from build123d import *

# Parameters (mm, degrees)
F0_W      = 5
F0_H      = 370
F1_DEPTH  = 100
F0_W_2    = 20
F0_W_3    = 389
F0_H_2    = 20
F2_DEPTH  = 5
F3_W      = 20
F3_H      = 370
F4_DEPTH  = 5
F3_W_2    = 389
F3_H_2    = 20
F5_DEPTH  = 5
F7_DEPTH  = 20
F8_DEPTH  = 25
F10_DEPTH = 20
F9_W      = 45
F9_H      = 5
F11_DEPTH = 100


with BuildPart() as f1:
    # F0 (on Front) → F1 (new body)
    with BuildSketch(Plane.XZ):
        Polygon((-205.3960859776, 18.3333333333), (-205.3960859776, 13.3333333333), (183.6039140224, 13.3333333333), (183.6039140224, 18.3333333333), (163.6039140225, 18.3333333333), (158.6039140225, 18.3333333333), (-180.3960859776, 18.3333333333), (-185.3960859776, 18.3333333333), align=None)
        with Locations((-182.8960859776, 203.3333333333)):
            Rectangle(F0_W, F0_H)
        with Locations((161.1039140225, 203.3333333333)):
            Rectangle(F0_W, F0_H)
    extrude(amount=F1_DEPTH)

    # F0 (on Front) → F2 (join)
    with BuildSketch(Plane.XZ):
        with Locations((-195.3960859776, 203.3333333333)):
            Rectangle(F0_W_2, F0_H)
        with Locations((-10.8960859776, 3.3333333333)):
            Rectangle(F0_W_3, F0_H_2)
        with Locations((173.6039140224, 203.3333333333)):
            Rectangle(F0_W_2, F0_H)
    extrude(amount=F2_DEPTH)

    # F3 (on face) → F4 (join)
    with BuildSketch(Plane.XZ.offset(100)):
        with Locations((-195.3960859776, 203.3333333333)):
            Rectangle(F3_W, F3_H)
    extrude(amount=-F4_DEPTH)

    # F3 (on face) → F5 (join)
    with BuildSketch(Plane.XZ.offset(100)):
        with Locations((-10.8960859776, 3.3333333333)):
            Rectangle(F3_W_2, F3_H_2)
        with Locations((173.6039140225, 203.3333333333)):
            Rectangle(F3_W, F3_H)
    extrude(amount=-F5_DEPTH)

    # F7 (cut): a face of the model
    f7_faces = [f1.faces().sort_by_distance(p)[0] for p in [
        (162.573137616, -50, 388.3333333333),
    ]]
    extrude(f7_faces, amount=-F7_DEPTH, mode=Mode.SUBTRACT)

    # F6 (on face) → F8 (cut)
    with BuildSketch(Plane.YZ.offset(-180.3960859776)):
        with BuildLine():
            Line((-81.7000014901, 341.2361545223), (-81.7000014901, 320.7823193073))
            Line((-81.7000014901, 320.7823193073), (-53.5750014901, 320.7823193073))
            ThreePointArc((-53.5750014901, 320.7823193073), (-51.7353107636, 325.2108260661), (-47.2992664142, 327.0322663236))
            Line((-47.2992664142, 327.0322663236), (-47.1841779607, 354.9823193073))
            Line((-47.1841779607, 354.9823193073), (-68.0701213982, 354.9823193073))
            ThreePointArc((-68.0701213982, 354.9823193073), (-75.7291590422, 348.9461939299), (-81.7000014901, 341.2361545223))
        make_face()
        with BuildLine():
            ThreePointArc((-81.7000014901, 341.2361545223), (-85.8931230415, 331.3889210251), (-87.3250014901, 320.7823193073))
            Line((-87.3250014901, 320.7823193073), (-81.7000014901, 320.7823193073))
            Line((-81.7000014901, 320.7823193073), (-81.7000014901, 341.2361545223))
        make_face()
        with BuildLine():
            Line((-81.7000014901, 320.7823193073), (-87.3250014901, 320.7823193073))
            ThreePointArc((-87.3250014901, 320.7823193073), (-85.8931230415, 310.1757175895), (-81.7000014901, 300.3284840924))
            Line((-81.7000014901, 300.3284840924), (-81.7000014901, 320.7823193073))
        make_face()
        with BuildLine():
            Line((-13.3000014901, 320.7823193073), (-13.3000014901, 299.7514045626))
            ThreePointArc((-13.3000014901, 299.7514045626), (-8.847735475, 309.8507137528), (-7.3250014901, 320.7823193073))
            ThreePointArc((-7.3250014901, 320.7823193073), (-8.847735475, 331.7139248619), (-13.3000014901, 341.8132340521))
            Line((-13.3000014901, 341.8132340521), (-13.3000014901, 320.7823193073))
        make_face()
        with BuildLine():
            Line((-47.3507365661, 314.5323722911), (-47.4658250195, 286.5823193073))
            Line((-47.4658250195, 286.5823193073), (-26.579881582, 286.5823193073))
            ThreePointArc((-26.579881582, 286.5823193073), (-19.1594603041, 292.3798143175), (-13.3000014901, 299.7514045626))
            Line((-13.3000014901, 299.7514045626), (-13.3000014901, 320.7823193073))
            Line((-13.3000014901, 320.7823193073), (-41.0750014901, 320.7823193073))
            ThreePointArc((-41.0750014901, 320.7823193073), (-42.9146922166, 316.3538125486), (-47.3507365661, 314.5323722911))
        make_face()
        with BuildLine():
            Line((-26.579881582, 354.9823193073), (-47.1841779607, 354.9823193073))
            Line((-47.1841779607, 354.9823193073), (-47.2992664142, 327.0322663236))
            ThreePointArc((-47.2992664142, 327.0322663236), (-42.8964947314, 325.1926285808), (-41.0750014901, 320.7823193073))
            Line((-41.0750014901, 320.7823193073), (-13.3000014901, 320.7823193073))
            Line((-13.3000014901, 320.7823193073), (-13.3000014901, 341.8132340521))
            ThreePointArc((-13.3000014901, 341.8132340521), (-19.1594603041, 349.1848242972), (-26.579881582, 354.9823193073))
        make_face()
        with BuildLine():
            Line((-53.5750014901, 320.7823193073), (-81.7000014901, 320.7823193073))
            Line((-81.7000014901, 320.7823193073), (-81.7000014901, 300.3284840924))
            ThreePointArc((-81.7000014901, 300.3284840924), (-75.7291590422, 292.6184446848), (-68.0701213982, 286.5823193073))
            Line((-68.0701213982, 286.5823193073), (-47.4658250195, 286.5823193073))
            Line((-47.4658250195, 286.5823193073), (-47.3507365661, 314.5323722911))
            ThreePointArc((-47.3507365661, 314.5323722911), (-51.7535082489, 316.3720100339), (-53.5750014901, 320.7823193073))
        make_face()
        with BuildLine():
            ThreePointArc((-68.0701213982, 286.5823193073), (-58.1746192575, 282.2818544491), (-47.4897059762, 280.7826584034))
            Line((-47.4897059762, 280.7826584034), (-47.4658250195, 286.5823193073))
            Line((-47.4658250195, 286.5823193073), (-68.0701213982, 286.5823193073))
        make_face()
        with BuildLine():
            Line((-47.4658250195, 286.5823193073), (-47.4897059762, 280.7826584034))
            ThreePointArc((-47.4897059762, 280.7826584034), (-36.6340056812, 282.237506315), (-26.579881582, 286.5823193073))
            Line((-26.579881582, 286.5823193073), (-47.4658250195, 286.5823193073))
        make_face()
        with BuildLine():
            Line((-47.3250014901, 320.7823193073), (-53.5750014901, 320.7823193073))
            ThreePointArc((-53.5750014901, 320.7823193073), (-51.7535082489, 316.3720100339), (-47.3507365661, 314.5323722911))
            Line((-47.3507365661, 314.5323722911), (-47.3250014901, 320.7823193073))
        make_face()
        with BuildLine():
            ThreePointArc((-47.2992664142, 327.0322663236), (-51.7353107636, 325.2108260661), (-53.5750014901, 320.7823193073))
            Line((-53.5750014901, 320.7823193073), (-47.3250014901, 320.7823193073))
            Line((-47.3250014901, 320.7823193073), (-47.2992664142, 327.0322663236))
        make_face()
        with BuildLine():
            Line((-47.2992664142, 327.0322663236), (-47.3250014901, 320.7823193073))
            Line((-47.3250014901, 320.7823193073), (-41.0750014901, 320.7823193073))
            ThreePointArc((-41.0750014901, 320.7823193073), (-42.8964947314, 325.1926285808), (-47.2992664142, 327.0322663236))
        make_face()
        with BuildLine():
            Line((-41.0750014901, 320.7823193073), (-47.3250014901, 320.7823193073))
            Line((-47.3250014901, 320.7823193073), (-47.3507365661, 314.5323722911))
            ThreePointArc((-47.3507365661, 314.5323722911), (-42.9146922166, 316.3538125486), (-41.0750014901, 320.7823193073))
        make_face()
        with BuildLine():
            Line((-47.1841779607, 354.9823193073), (-47.160297004, 360.7819802113))
            ThreePointArc((-47.160297004, 360.7819802113), (-58.015997299, 359.3271322997), (-68.0701213982, 354.9823193073))
            Line((-68.0701213982, 354.9823193073), (-47.1841779607, 354.9823193073))
        make_face()
        with BuildLine():
            ThreePointArc((-26.579881582, 354.9823193073), (-36.4753837227, 359.2827841656), (-47.160297004, 360.7819802113))
            Line((-47.160297004, 360.7819802113), (-47.1841779607, 354.9823193073))
            Line((-47.1841779607, 354.9823193073), (-26.579881582, 354.9823193073))
        make_face()
    extrude(amount=-F8_DEPTH, mode=Mode.SUBTRACT)

    # F10 (cut): a face of the model
    f10_faces = [f1.faces().sort_by_distance(p)[0] for p in [
        (-204.3653095712, -2.5, 388.3333333333),
    ]]
    extrude(f10_faces, amount=-F10_DEPTH, mode=Mode.SUBTRACT)

    # F9 (on face) → F11 (join)
    with BuildSketch(Plane(origin=(-185.3960859776, 0, 0), x_dir=(0, -1, 0), z_dir=(-1, 0, 0))):
        with Locations((72.5, 54.8333333333)):
            Rectangle(F9_W, F9_H)
        with Locations((27.5, 54.8333333333)):
            Rectangle(F9_W, F9_H)
    extrude(amount=F11_DEPTH)


solid = f1.part
CAD build for the part. Positions are in the model's coordinates, mm. A direction names the side the tool comes from. Coordinates: 2 decimals unless noted, no trailing zeros. Order: outer loops, then holes, each group sorted by start corner. A loop starts at its lowest first (then second) coordinate and runs counter-clockwise, first axis right, second up. Notation, with made-up numbers: (-39.75, 87.25) -> (-6.75, 87.25) arc R12 ccw to (-6.75, 95.25) -> close; hole circle Ø6 at (22, -7.5). An arc over 180 degrees is marked (long way). Answer in a Markdown table with one row per item.
1) Flat gauge pins, fed straight in: P1, Ø2, axis at x = -32, y = -51.5, coming from the -Z side; P2, Ø17, axis at y = -53.5, z = 31.5, coming from the -X side; P3, Ø16, axis at x = 176, y = -39, coming from the +Z side. Where does each tip first touch, or does it go through?
Check values:
| item | result |
|---|---|
| P1 | z = 13.33 |
| P2 | x = -185.4 |
| P3 | z = 18.33 |
2) Band-saw the part on D-D (x = -5.5). List the corners of the cut face in (y, z), and give its area (3 significant figures).
Check values:
| item | result |
|---|---|
| outline | (-100, -6.67) -> (-95, -6.67) -> (-95, 13.33) -> (-5, 13.33) -> (-5, -6.67) -> (0, -6.67) -> (0, 18.33) -> (-100, 18.33) -> close |
| area | 700 mm2 |
3) Band-saw the part on C-C (y = -61). List the corners of the cut face in (x, z).
Check values:
| item | result |
|---|---|
| outline | (-285.4, 52.33) -> (-185.4, 52.33) -> (-185.4, 18.33) -> (-205.4, 18.33) -> (-205.4, 13.33) -> (183.6, 13.33) -> (183.6, 18.33) -> (163.6, 18.33) -> (163.6, 368.33) -> (158.6, 368.33) -> (158.6, 18.33) -> (-180.4, 18.33) -> (-180.4, 283.19) -> (-185.4, 283.19) -> (-185.4, 57.33) -> (-285.4, 57.33) -> close; (-185.4, 358.37) -> (-180.4, 358.37) -> (-180.4, 368.33) -> (-185.4, 368.33) -> close |
4) Which spindle directions (+Z, -Z, +X, -X, +Y, -Y) get a long thin tool onto all of the face, cutting with end or side? Do faces 1 (the face through (-14, -49, 13.333)), 2 (the face through (-196, -5, 36)), 3 (the face through (173, -95, 196)), 4 (the face through (-196, -5, 215)), 5 (the face through (-9, -49, 18.333)). Say none if no direction does.
Check values:
| item | result |
|---|---|
| face 1 | -Z, +X, -X |
| face 2 | -X |
| face 3 | +Z, +X |
| face 4 | +Z, -X |
| face 5 | +Z, +Y, -Y |
5) Band-saw the part on A-A (z = 77.5). List the corners of the cut face in (x, y), and give its area (3 significant figures).
Check values:
| item | result |
|---|---|
| outline | (-205.4, -100) -> (-180.4, -100) -> (-180.4, 0) -> (-205.4, 0) -> (-205.4, -5) -> (-185.4, -5) -> (-185.4, -95) -> (-205.4, -95) -> close; (158.6, -100) -> (183.6, -100) -> (183.6, -95) -> (163.6, -95) -> (163.6, -5) -> (183.6, -5) -> (183.6, 0) -> (158.6, 0) -> close |
| area | 1,400 mm2 |
6) Drill centre lines: line 1 (X direction, y = -56, z = 263.5); line 2 (Z direction, x = -203.5, y = -69); line 3 (X direction, y = -36, z = 57). Where is each one in solid material? Low to high.
Check values:
| item | result |
|---|---|
| line 1 | -185.4 to -180.4, 158.6 to 163.6 |
| line 2 | 13.33 to 18.33, 52.33 to 57.33 |
| line 3 | -285.4 to -180.4, 158.6 to 163.6 |
7) Band-saw the part on B-B (x = -190.5). List the corners of the cut face in (y, z), and give its area (3 significant figures).
Check values:
| item | result |
|---|---|
| outline | (-100, -6.67) -> (-95, -6.67) -> (-95, 13.33) -> (-5, 13.33) -> (-5, -6.67) -> (0, -6.67) -> (0, 368.33) -> (-5, 368.33) -> (-5, 57.33) -> (-95, 57.33) -> (-95, 368.33) -> (-100, 368.33) -> close; hole (-95, 18.33) -> (-5, 18.33) -> (-5, 52.33) -> (-95, 52.33) -> close |
| area | 4,650 mm2 |
8) Mould opens along X. For faces 6 (the face through (158.604, -49, 191)), 7 (the face through (-195, -49, 18.333)), 8 (the face through (-185.396, -49, 35)) say: pulls with the +X half, pulls with the -X half, needs draft (parallel to the pull), parting line crosses it, or undercut.
Check values:
| item | result |
|---|---|
| face 6 | undercut |
| face 7 | needs draft |
| face 8 | pulls with the -X half |
